Here's the drawing with two shaded views (mm, measured from the low corner). I have some questions. A direction names the side the tool comes from. Coordinates: 2 decimals unless noted, no trailing zeros. Write each loop counter-clockwise with the first axis right and the second up, starting at its lowest first coordinate (ties: lowest second). Pieces come first, ordered by that corner, then holes. Notation, with made-up numbers: (66.25, 65) -> (118.25, 65) arc R16 cw to (118.25, 71) -> close; hole circle Ø9 at (-19.75, 73.25). An arc over 180 degrees is marked (long way). Put each result on its own line as item: value. Start each with the question number.
Item 1: On a 3-axis mill with a long thin cutter (end or side, diameter ignored), from which of +Z, -Z, +X, -X, +Y, -Y can I reach the whole of each face in a straight line? I mean the marked faces 1 and 2. Say none if no direction works.
Item 2: I want a section at C-C, the plane y = 4.75. List the corners of the cut face in (x, z) for me.
Item 3: For pin 1 (3 mm diameter, centred on y = 5.5, z = 19, fed in from -X); pin 2 (4 mm diameter, centred on x = 6.5, y = 5, fed in from -Z); pin 3 (8 mm diameter, centred on x = 10, y = 16.5, fed in from +Z); pin 4 (10.5 mm diameter, centred on x = 11.5, z = 20.5, fed in from -Y), each with a flat end and sliding along its axis, tell me the tip position at first contact or that it passes through.
Item 4: I want a section at A-A, the plane z = 17.5. List the corners of the cut face in (x, y) for me.
Item 5: I want a section at B-B, the plane x = 17.5. List the corners of the cut face in (y, z) for me.
Item 6: I need wall thicknesses on line 1 (Y direction, x = 21.5, z = 2); line 2 (X direction, y = 6, z = 17); line 3 (X direction, y = 23.75, z = 32). Which ranges of each line are inside material? Lowest first, please. Write a range as [from, to].
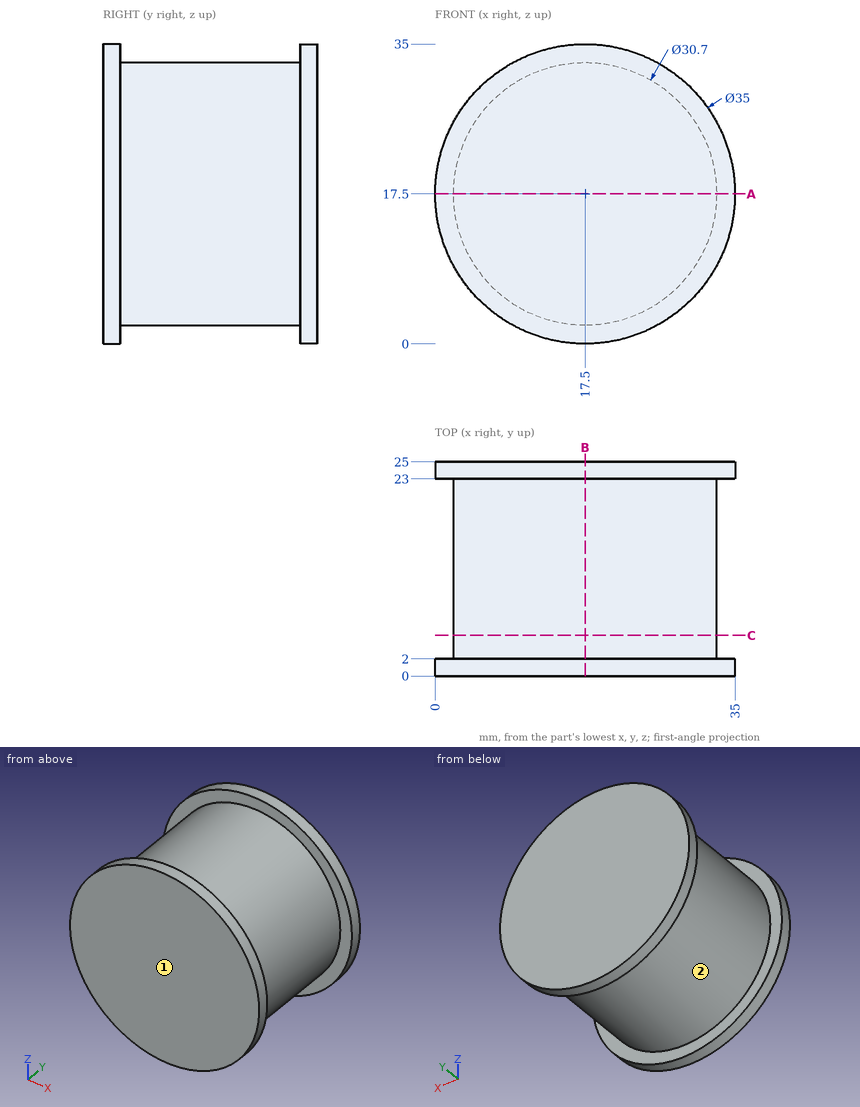
Calculated:
1. face 1: +Z, -Z, +X, -X, -Y
1. face 2: none
2. outline: circle Ø30.7 at (17.5, 17.5)
3. pin 1: stops at x = 2.15
3. pin 2: stops at z = 5.07
3. pin 3: stops at z = 32.45
3. pin 4: stops at y = 0
4. outline: (0, 0) -> (35, 0) -> (35, 2) -> (32.85, 2) -> (32.85, 23) -> (35, 23) -> (35, 25) -> (0, 25) -> (0, 23) -> (2.15, 23) -> (2.15, 2) -> (0, 2) -> close
5. outline: (0, 0) -> (2, 0) -> (2, 2.15) -> (23, 2.15) -> (23, 0) -> (25, 0) -> (25, 35) -> (23, 35) -> (23, 32.85) -> (2, 32.85) -> (2, 35) -> (0, 35) -> close
6. line 1: y = [0, 2], [23, 25]
6. line 2: x = [2.16, 32.84]
6. line 3: x = [7.7, 27.3]
